```python
from build123d import *

# Parameters (mm, degrees)
SKETCH1_W           = 152.4
SKETCH1_H           = 152.4
BOSS_EXTRUDE1_DEPTH = 10.16
SKETCH3_R           = 38.1
BOSS_EXTRUDE3_DEPTH = 12.7
SKETCH4_R           = 4
BOSS_EXTRUDE4_DEPTH = 18
SKETCH7_R           = 3.175
CUT_EXTRUDE2_DEPTH  = 10.16


with BuildPart() as part:
    # Sketch1 → Boss-Extrude1 (new body)
    with BuildSketch(Plane(origin=(0, 0, 0), x_dir=(1, 0, 0), z_dir=(0, 1, 0))):
        Rectangle(SKETCH1_W, SKETCH1_H)
    extrude(amount=BOSS_EXTRUDE1_DEPTH)

    # Sketch3 → Boss-Extrude3 (add)
    with BuildSketch(Plane.XZ):
        with Locations(Location((0, 0, 0), (0, 0, 270))):
            Circle(SKETCH3_R)
    extrude(amount=BOSS_EXTRUDE3_DEPTH)

    # Sketch4 → Boss-Extrude4 (add)
    with BuildSketch(Plane.XZ.offset(12.7)):
        with Locations(Location((0, 0, 0), (0, 0, 270))):
            Circle(SKETCH4_R)
    extrude(amount=BOSS_EXTRUDE4_DEPTH)

    # Sketch7 → Cut-Extrude2 (cut)
    with BuildSketch(Plane(origin=(0, 10.16, 0), x_dir=(1, 0, 0), z_dir=(0, 1, 0))):
        with Locations(Location((-41.57222955, 26.925278647, 0), (0, 0, 270))):
            Circle(SKETCH7_R)
        with Locations(Location((-2.531860538, 49.465246206, 0), (0, 0, 270))):
            Circle(SKETCH7_R)
        with Locations(Location((-6.594762938, -49.089000823, 0), (0, 0, 270))):
            Circle(SKETCH7_R)
        with Locations(Location((45.809703228, -18.833268175, 0), (0, 0, 270))):
            Circle(SKETCH7_R)
    extrude(amount=-CUT_EXTRUDE2_DEPTH, mode=Mode.SUBTRACT)


solid = part.part
```
Geometry: final body of the model. Coordinates: model frame, mm. A direction names the side the tool comes from. Round coordinates to 2 decimals unless told otherwise and drop trailing zeros. Order: outer loops, then holes, each group sorted by start corner. A loop starts at its lowest first (then second) coordinate and runs counter-clockwise, first axis right, second up. Notation, with made-up numbers: (33.5, 63) - (40.5, 63) arc R21 ccw to (40.5, 77) - close; hole circle Ø2 at (48, 67). An arc over 180 degrees is marked (long way). Write item = value, one per line. Start each with the question number.
Q1. Cut plane B-B on y = -17. Return the cut outline in (x, z), and give its area (3 significant figures).
Q2. Cut plane D-D on y = -2. Return the cut outline in (x, z).
Q3. Cut plane A-A on z = 0. Return the cut outline in (x, y).
Q4. Access query for faces 5 (the cylindrical face through (-6.455, 5.151, 45.917)), 6 (the cylindrical face through (-3.905, -21.574, 0.867)). Directions: +Z, -Z, +X, -X, +Y, -Y. A direction counts if a zero-diameter tool reaches every point of the face in a straight line with its end or side. Return the directions, or none.
Q5. Pin query (flat end, axial travel): pin 1 (8 mm diameter, centred on x = 31, y = -12, fed in from +Z); pin 2 (6 mm diameter, centred on x = -24, y = -13.5, fed in from -Z); pin 3 (23 mm diameter, centred on x = -14.5, z = -13.5, fed in from -Y); pin 4 (10 mm diameter, centred on x = -6.59, z = 49.09, fed in from +Y). Return the tip coordinate at first contact, or that it passes through.
Q6. Pull-direction query (X, two-part tool) for faces 1 (the flat face through (-1, 5, 76.2)), 2 (the cylindrical face through (48.487, 5.151, 20.54)), 3 (the flat face through (76.2, 5, 1)), 4 (the cylindrical face through (-1.578, 5.151, -46.437)); classes: +X half, -X half, draft (parallel to the pull), parting line (faces both ways), or undercut.
Q7. Cut plane C-C on x = 34.5. Return the cut outline in (y, z), and give its area (3 significant figures).
Q8. Ray query, line 1 (X direction, y = 4.5, z = -27); line 2 (Y direction, x = -69.5, z = 11); line 3 (Y direction, x = 12, z = 18). Return the intervals inside material, ascending. Write a range as from..to.
Outcome:
q1.outline = circle Ø8 at (0, 0)
q1.area = 50.3 mm^2
q2.outline = circle Ø76.2 at (0, 0)
q3.outline = (-76.2, 0) - (-38.1, 0) - (-38.1, -12.7) - (-4, -12.7) - (-4, -30.7) - (4, -30.7) - (4, -12.7) - (38.1, -12.7) - (38.1, 0) - (76.2, 0) - (76.2, 10.16) - (-76.2, 10.16) - close
q4.face_5 = +Y, -Y
q4.face_6 = -Y
q5.pin_1 = 26.88
q5.pin_2 = -31.72
q5.pin_3 = -12.7
q5.pin_4 = 10.16
q6.face_1 = draft
q6.face_2 = undercut
q6.face_3 = +X half
q6.face_4 = undercut
q7.outline = (-12.7, -16.17) - (0, -16.17) - (0, -76.2) - (10.16, -76.2) - (10.16, 76.2) - (0, 76.2) - (0, 16.17) - (-12.7, 16.17) - close
q7.area = 1,960 mm^2
q8.line_1 = -76.2..-44.75, -38.4..76.2
q8.line_2 = 0..10.16
q8.line_3 = -12.7..10.16
